from build123d import *

# Parameters (mm, degrees)
F4_DEPTH = 7


with BuildPart() as f4:
    # F0 (on Top) → F4 (new body)
    with BuildSketch(Plane.XY):
        Polygon((175, -101.0362971082), (0, 202.0725942164), (-175, -101.0362971082), align=None)
    extrude(amount=-F4_DEPTH)

    # F3: sweep along a path in F2
    with BuildLine(Plane.XY) as f3_path:
        Line((-149.1875, -86.1334432847), (149.1875, -86.1334432847))
        Line((149.1875, -86.1334432847), (0, 172.2668865695))
        Line((0, 172.2668865695), (-149.1875, -86.1334432847))
    # F1 (on Right) → F3 (sweep, cut)
    with BuildSketch(Plane.YZ):
        Polygon((-86.8137743667, -3.5), (-86.1334432847, 0), (-89.4442725433, 0), (-90.1246036253, -3.5), align=None)
    sweep(path=f3_path.line, transition=Transition.RIGHT, mode=Mode.SUBTRACT)


solid = f4.part
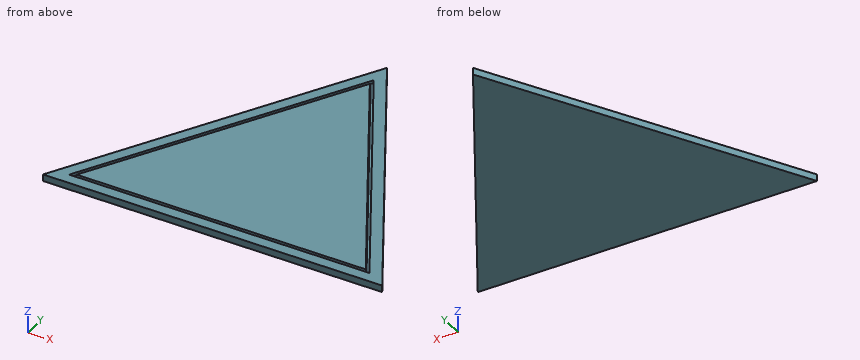
Check sheet for the modelled part. Datum: model origin and axes. Units: mm. Round coordinates to 2 decimals unless told otherwise and drop trailing zeros. Loops run counter-clockwise (first coordinate to the right, second up) from the corner with the lowest first, then second, coordinate; pieces in that order, holes last. Notation, with made-up numbers: M -22,36.5 L 12,36.5 A18 cw 12,54.5 Z; hole C 18.5,-6.75 d11. An arc over 180 degrees is marked long. One line per item, written item: value.
(1) Thickness scan on line 1 (Y direction, x = 46.5, z = -1); line 2 (X direction, y = 57, z = -1); line 3 (X direction, y = 69, z = -1.25). Record the ranges inside material, lowest first.
Computed values:
line 1: y = -101.04 to -89.64, -86.33 to 92.12, 98.74 to 121.53
line 2: x = -83.76 to -70.6, -66.77 to 66.77, 70.6 to 83.76
line 3: x = -76.83 to -63.72, -59.9 to 59.9, 63.72 to 76.83
(2) Depth check by flat-ended pin: pin 1 Ø1 at (y, z) = (-43, -3.5) entering from -X. Enter the tip coordinate at first touch or a pass-through.
Computed values:
pin 1: stops at x = -141.78
(3) Sectioned sample at B-B, the plane x = 134.5. Record the cut outline in (y, z).
Computed values:
outline: M -101.04,-7 L -30.89,-7 L -30.89,0 L -54.07,0 L -52.71,-3.5 L -59.33,-3.5 L -60.69,0 L -86.13,0 L -86.81,-3.5 L -90.12,-3.5 L -89.44,0 L -101.04,0 Z
(4) Sectioned sample at C-C, the plane y = -21. Record the cut outline in (x, z).
Computed values:
outline: M -128.79,-7 L 128.79,-7 L 128.79,0 L 115.41,0 L 116.19,-3.5 L 112.37,-3.5 L 111.58,0 L -111.58,0 L -112.37,-3.5 L -116.19,-3.5 L -115.41,0 L -128.79,0 Z
(5) Sectioned sample at A-A, the plane z = -1.25. Record the cut outline in (x, y), then the cut area to 3 significant figures.
Computed values:
outline: M -175,-101.04 L 175,-101.04 L 0,202.07 Z; M -149.61,-86.38 L 149.61,-86.38 L 0,172.75 Z; hole M -155.34,-89.69 L 155.34,-89.69 L 0,179.37 Z
area: 50,000 mm^2
